Input: dimensioned drawing with shaded views. Units: mm. Origin: part minimum x, y, z. Give positions to 0.01 mm unless a question says otherwise; leave off trailing zeros. Write each loop counter-clockwise with the first axis right and the second up, starting at its lowest first coordinate (ties: lowest second). Pieces come first, ordered by that corner, then holes.
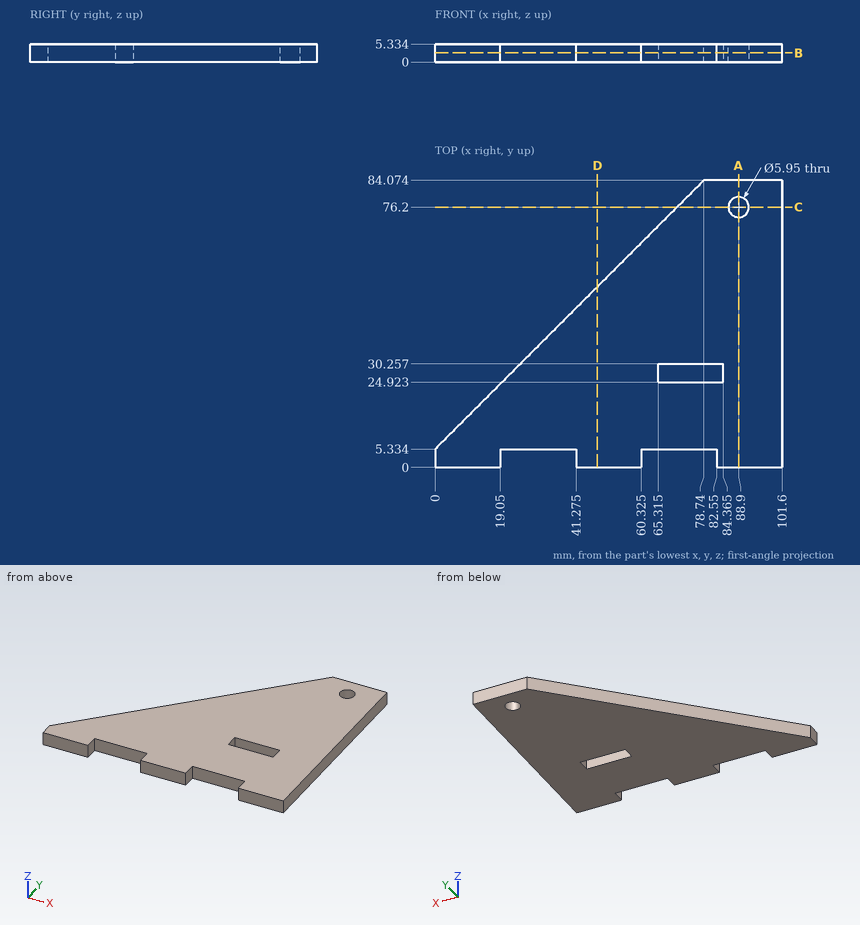
1. Line query: L1, parallel to Y at x = 88.9, z = 4.1 (1 decimal); L2, parallel to X at y = 27, z = 1.15 (1 decimal); L3, parallel to Y at x = 70, z = 4.5 (1 decimal). Output: solid intervals per line, ascending.
2. Contact query for flat-ended pins moving along their axis: P1, Ø1.5, axis at x = 51.5, z = 1.5, coming from the +Y side (1 decimal); P2, Ø2.5, axis at x = 29, z = 3, coming from the -Y side; P3, Ø1, axis at x = 39, z = 4.5, coming from the +Y side (1 decimal). Output: stop coordinate, or through.
3. Cut plane B-B, the plane z = 2.75. State how many separate pieces and enclosed holes the cut face has, then the cut area to 3 significant figures.
4. Cut plane A-A, the plane x = 88.9. Return the cut outline in (y, z) (1 decimal), then the cut area to 3 significant figures.
5. Cut plane D-D, the plane x = 47.5. Return the cut outline in (y, z), then the cut area to 3 significant figures.
6. Cut plane C-C, the plane y = 76.2. Return the cut outline in (x, z) (1 decimal).
Response values:
1. L1: y = 0 to 73.2, 79.2 to 84.1
1. L2: x = 21.7 to 65.3, 84.4 to 101.6
1. L3: y = 5.3 to 24.9, 30.3 to 75.3
2. P1: stops at y = 57.6
2. P2: stops at y = 5.33
2. P3: stops at y = 44.8
3. separate pieces: 1
3. enclosed holes: 2
3. area: 5,080 mm2
4. outline: (0, 0) - (73.2, 0) - (73.2, 5.3) - (0, 5.3) - close; (79.2, 0) - (84.1, 0) - (84.1, 5.3) - (79.2, 5.3) - close
4. area: 417 mm2
5. outline: (0, 0) - (52.83, 0) - (52.83, 5.33) - (0, 5.33) - close
5. area: 282 mm2
6. outline: (70.9, 0) - (85.9, 0) - (85.9, 5.3) - (70.9, 5.3) - close; (91.9, 0) - (101.6, 0) - (101.6, 5.3) - (91.9, 5.3) - close
